The listing builds one solid part. Answer for the finished solid, in the listing's coordinates (mm). A direction names the side the tool comes from. Coordinates: 2 decimals unless noted, no trailing zeros. Write each loop counter-clockwise with the first axis right and the second up, starting at its lowest first coordinate (ties: lowest second). Pieces come first, ordered by that corner, then holes.
```python
from build123d import *

# Parameters (mm, degrees)
F0_W      = 59
F0_H      = 84
F0_R      = 1.5
F1_DEPTH  = 2
F2_W      = 40
F2_H      = 40
F3_DEPTH  = 12
F4_W      = 18
F4_H      = 13
F5_DEPTH  = 16
F6_W      = 13
F6_H      = 5
F7_DEPTH  = 30
F8_W      = 10
F8_H      = 8
F9_DEPTH  = 10
F10_R     = 4
F11_DEPTH = 15
F12_W     = 11
F12_H     = 15
F13_DEPTH = 6
F14_W     = 15
F14_H     = 6
F15_DEPTH = 15


with BuildPart() as f1:
    # F0 (on Top) → F1 (new body)
    with BuildSketch(Plane.XY):
        Rectangle(F0_W, F0_H)
        with Locations((-26, -38)):
            Circle(F0_R, mode=Mode.SUBTRACT)
        with Locations((26, -38)):
            Circle(F0_R, mode=Mode.SUBTRACT)
        with Locations((-26, 38)):
            Circle(F0_R, mode=Mode.SUBTRACT)
        with Locations((26, 38)):
            Circle(F0_R, mode=Mode.SUBTRACT)
    extrude(amount=F1_DEPTH)

    # F2 (on face) → F3 (join)
    with BuildSketch(Plane.XY.offset(2)):
        with Locations((-2, 14)):
            Rectangle(F2_W, F2_H)
    extrude(amount=F3_DEPTH)

    # F4 (on face) → F5 (join)
    with BuildSketch(Plane.XY.offset(2)):
        with Locations((-20.5, -27.5)):
            Rectangle(F4_W, F4_H)
    extrude(amount=F5_DEPTH)

    # F6 (on face) → F7 (join)
    with BuildSketch(Plane(origin=(-29.5, 0, 0), x_dir=(0, -1, 0), z_dir=(-1, 0, 0))):
        with Locations((27.5, 15.5)):
            Rectangle(F6_W, F6_H)
        with Locations((27.5, 7.5)):
            Rectangle(F6_W, F6_H)
    extrude(amount=F7_DEPTH)

    # F8 (on face) → F9 (join)
    with BuildSketch(Plane.XY.offset(2)):
        with Locations((24.5, -1)):
            Rectangle(F8_W, F8_H)
    extrude(amount=F9_DEPTH)

    # F10 (on face) → F11 (join)
    with BuildSketch(Plane.YZ.offset(29.5)):
        with Locations((-1, 8)):
            Circle(F10_R)
    extrude(amount=F11_DEPTH)

    # F12 (on face) → F13 (join)
    with BuildSketch(Plane.XY.offset(2)):
        with Locations((24, 26.5)):
            Rectangle(F12_W, F12_H)
    extrude(amount=F13_DEPTH)

    # F14 (on face) → F15 (join)
    with BuildSketch(Plane.YZ.offset(29.5)):
        with Locations((26.5, 5)):
            Rectangle(F14_W, F14_H)
    extrude(amount=F15_DEPTH)


solid = f1.part
```
(1) Each of these flat-tipped pins is pushed along its axis until it touches: pin 1 (3 mm diameter, centred on x = 27.5, z = 6.5, fed in from -Y); pin 2 (1.5 mm diameter, centred on x = -21.5, y = 7, fed in from +Z); pin 3 (6.5 mm diameter, centred on y = 25, z = 6.5, fed in from -X). Where does it stop, or does it pass through?
(2) Section A-A, the plane x = 26 is taken. Write down the section's boundary in (y, z).
(3) Section C-C, the plane x = -44 is taken. Write down the section's boundary in (y, z).
(4) Which of the six approach directions +Z, -Z, +X, -X, +Y, -Y give full straight-line access (tool end or side, diameter ignored) to faces 4 (the flat face through (-44, -27, 5)), 5 (the flat face through (31, 19, 5)), 6 (the flat face through (29.5, 2, 11)), 7 (the flat face through (-35.2, -21, 13.4))?
(5) Find the intervals of material crossed by probe 1 along Y at (x, z) = (-26, 0.55); probe 2 along Y at (x, z) = (-15.5, 10); probe 3 along Y at (x, z) = (-0.5, 6.75), in increasing order.
(6) Section D-D, the plane y = -23.5 is taken. Write down the section's boundary in (x, z).
(7) Section B-B, the plane y = -38 is taken. Write down the section's boundary in (x, z).
(8) For a pull along X with two mould halves and no side action, classify faces 1 (the cylindrical face through (-27.2, -38.9, 1)), 2 (the flat face through (-59.5, -27, 8)), 3 (the flat face through (24, 3, 7)) as pulls with the +X half, pulls with the -X half, needs draft (parallel to the pull), parting line crosses it, or undercut.
Solution:
1. pin 1: stops at y = -5
1. pin 2: stops at z = 14
1. pin 3: stops at x = -22
2. outline: (-42, 0) - (-39.5, 0) - (-39.5, 2) - (-42, 2) - close; (-36.5, 0) - (36.5, 0) - (36.5, 2) - (34, 2) - (34, 8) - (19, 8) - (19, 2) - (3, 2) - (3, 12) - (-5, 12) - (-5, 2) - (-36.5, 2) - close; (39.5, 0) - (42, 0) - (42, 2) - (39.5, 2) - close
3. outline: (-34, 5) - (-21, 5) - (-21, 10) - (-34, 10) - close; (-34, 13) - (-21, 13) - (-21, 18) - (-34, 18) - close
4. face 4: -Z, -X, +Y, -Y
4. face 5: +Z, +X
4. face 6: +Z, +X, +Y
4. face 7: +Z, +X, -X
5. probe 1: y = -42 to -39.5, -36.5 to 36.5, 39.5 to 42
5. probe 2: y = -34 to -21, -6 to 34
5. probe 3: y = -6 to 34
6. outline: (-59.5, 5) - (-29.5, 5) - (-29.5, 0) - (29.5, 0) - (29.5, 2) - (-11.5, 2) - (-11.5, 18) - (-59.5, 18) - (-59.5, 13) - (-29.5, 13) - (-29.5, 10) - (-59.5, 10) - close
7. outline: (-29.5, 0) - (-27.5, 0) - (-27.5, 2) - (-29.5, 2) - close; (-24.5, 0) - (24.5, 0) - (24.5, 2) - (-24.5, 2) - close; (27.5, 0) - (29.5, 0) - (29.5, 2) - (27.5, 2) - close
8. face 1: undercut
8. face 2: pulls with the -X half
8. face 3: needs draft
